from build123d import *

# Parameters (mm, degrees)
BOSS_EXTRUDE1_DEPTH              = 5
MAINSKETCH_19_W                  = 18
MAINSKETCH_19_H                  = 18
BOSS_EXTRUDE2_DEPTH              = 5
CUT_EXTRUDE1_START               = 9
SKETCH1_R                        = 2.5
CUT_EXTRUDE1_DEPTH               = 13
SKETCH2_W                        = 1
SKETCH2_H                        = 3
CUT_EXTRUDE2_DEPTH               = 6
MIRROR2_COPY_1_SKETCH_W          = 1
MIRROR2_COPY_1_SKETCH_H          = 3
MIRROR2_COPY_1_DEPTH             = 6
HOLESKETCH_R                     = 4
CUT_EXTRUDE3_DEPTH               = 6
CUT_EXTRUDE3_DEPTH_BACK          = 2
CUT_EXTRUDE4_DEPTH               = 3
SCHNITT_LINEAR_AUSTRAGEN2_DEPTH  = 2.5
SKIZZE3_R                        = 1.75
SCHNITT_LINEAR_AUSTRAGEN3_DEPTH  = 11
SKIZZE4_R                        = 1.75
SCHNITT_LINEAR_AUSTRAGEN4_DEPTH  = 1.5
SKIZZE6_R                        = 1.75
SCHNITT_LINEAR_AUSTRAGEN6_DEPTH  = 11
SKIZZE7_R                        = 1.75
SCHNITT_LINEAR_AUSTRAGEN7_DEPTH  = 2.5
SKIZZE8_R                        = 1.75
SCHNITT_LINEAR_AUSTRAGEN8_DEPTH  = 11
SKIZZE9_R                        = 1.75
SCHNITT_LINEAR_AUSTRAGEN10_DEPTH = 2.5


with BuildPart() as part:
    # mainSketch → Boss-Extrude1 (new body)
    with BuildSketch(Plane(origin=(0, 0, 0), x_dir=(1, 0, 0), z_dir=(0, 1, 0))):
        with BuildLine():
            ThreePointArc((-18.215390309, 53), (-32.07179677, 53), (-39, 41))
            Line((-39, 41), (-39, -41))
            ThreePointArc((-39, -41), (-32.07179677, -53), (-18.215390309, -53))
            Line((-18.215390309, -53), (31.145825623, -24.501288694))
            ThreePointArc((31.145825623, -24.501288694), (45.291651246, 0), (31.145825623, 24.501288694))
            Line((31.145825623, 24.501288694), (-18.215390309, 53))
        make_face()
        Polygon((-9, -13.55), (-9, 4.45), (-9, 8.45), (9, 8.45), (9, 4.45), (9, -13.55), (9, -17.55), (-9, -17.55), align=None, mode=Mode.SUBTRACT)
    extrude(amount=BOSS_EXTRUDE1_DEPTH)

    # mainSketch_19 → Boss-Extrude2 (add)
    with BuildSketch(Plane(origin=(0, 0, 0), x_dir=(1, 0, 0), z_dir=(0, 1, 0))):
        with BuildLine():
            ThreePointArc((-18.215390309, 53), (-32.07179677, 53), (-39, 41))
            Line((-39, 41), (-39, -41))
            ThreePointArc((-39, -41), (-32.07179677, -53), (-18.215390309, -53))
            Line((-18.215390309, -53), (31.145825623, -24.501288694))
            ThreePointArc((31.145825623, -24.501288694), (45.291651246, 0), (31.145825623, 24.501288694))
            Line((31.145825623, 24.501288694), (-18.215390309, 53))
        make_face()
        with Locations((0, -4.55)):
            Rectangle(MAINSKETCH_19_W, MAINSKETCH_19_H, mode=Mode.SUBTRACT)
    extrude(amount=-BOSS_EXTRUDE2_DEPTH)

    # Sketch1 → Cut-Extrude1 (cut, symmetric)
    with BuildSketch(Plane(origin=(0, 0, 13.55), x_dir=(-1, 0, 0), z_dir=(0, 0, -1)).offset(CUT_EXTRUDE1_START)):
        Circle(SKETCH1_R)
    extrude(amount=CUT_EXTRUDE1_DEPTH, both=True, mode=Mode.SUBTRACT)

    # Sketch2 → Cut-Extrude2 (cut, through all)
    with BuildSketch(Plane(origin=(0, 0, 0), x_dir=(1, 0, 0), z_dir=(0, 1, 0))):
        with Locations((5, -15.55)):
            Rectangle(SKETCH2_W, SKETCH2_H)
    cut_extrude2 = extrude(amount=-CUT_EXTRUDE2_DEPTH, mode=Mode.SUBTRACT)

    # Mirror1: Cut-Extrude2 across plane
    add(cut_extrude2.mirror(Plane(origin=(0, 0, 0), x_dir=(0, 0, 1), z_dir=(1, 0, 0))), mode=Mode.SUBTRACT)

    # Mirror2: Cut-Extrude2 across plane
    add(cut_extrude2.mirror(Plane(origin=(0, 0, 4.55), x_dir=(1, 0, 0), z_dir=(0, 0, -1))), mode=Mode.SUBTRACT)

    # Mirror2 copy 1 sketch → Mirror2 copy 1 (cut, through all)
    with BuildSketch(Plane(origin=(0, 0, 9.1), x_dir=(-1, 0, 0), z_dir=(0, 1, 0))):
        with Locations((5, -15.55)):
            Rectangle(MIRROR2_COPY_1_SKETCH_W, MIRROR2_COPY_1_SKETCH_H)
    extrude(amount=-MIRROR2_COPY_1_DEPTH, mode=Mode.SUBTRACT)

    # holeSketch → Cut-Extrude3 (cut, two sides)
    with BuildSketch(Plane.XZ) as cut_extrude3_sk:
        with Locations(Location((29.25, -15.5, 0), (0, 0, 270))):  # turned: the seam where the file's is
            Circle(HOLESKETCH_R)
        with Locations(Location((-2.443479184, 27.5, 0), (0, 0, 270))):  # turned: the seam where the file's is
            Circle(HOLESKETCH_R)
        with Locations(Location((-29.6, -18.5, 0), (0, 0, 270))):  # turned: the seam where the file's is
            Circle(HOLESKETCH_R)
    extrude(amount=CUT_EXTRUDE3_DEPTH, mode=Mode.SUBTRACT)
    extrude(cut_extrude3_sk.sketch, amount=-CUT_EXTRUDE3_DEPTH_BACK, mode=Mode.SUBTRACT)

    # Sketch3 → Cut-Extrude4 (cut, symmetric)
    with BuildSketch(Plane(origin=(0, 0, 0), x_dir=(1, 0, 0), z_dir=(0, 1, 0))):
        with BuildLine():
            Line((-29.6, 26.5), (-39, 26.5))
            Line((-39, 26.5), (-39.6, 26.5))
            Line((-39.6, 26.5), (-39.6, -6.5))
            Line((-39.6, -6.5), (-37.6, -6.5))
            Line((-37.6, -6.5), (-21.6, -6.5))
            Line((-21.6, -6.5), (-21.6, 18.5))
            ThreePointArc((-21.6, 18.5), (-23.943145751, 24.156854249), (-29.6, 26.5))
        make_face()
        with BuildLine():
            Line((4.484724046, -23.5), (11.583570163, -35.79556215))
            Line((11.583570163, -35.79556215), (-8.960116539, -56.33889432))
            Line((-8.960116539, -56.33889432), (-14.464495813, -50.834420053))
            Line((-14.464495813, -50.834420053), (-25.778106688, -39.520613931))
            Line((-25.778106688, -39.520613931), (-8.100284622, -21.843096939))
            ThreePointArc((-8.100284622, -21.843096939), (-1.399235427, -19.568445614), (4.484724046, -23.5))
        make_face()
        with BuildLine():
            Line((40.858217841, 16.978745932), (35.413092194, 10.399382918))
            ThreePointArc((35.413092194, 10.399382918), (30.548118213, 7.606021972), (25.044818187, 8.694381298))
            Line((25.044818187, 8.694381298), (3.777259743, 21.835574464))
            Line((3.777259743, 21.835574464), (12.187623369, 35.446811868))
            Line((12.187623369, 35.446811868), (14.338041609, 38.927024434))
            Line((14.338041609, 38.927024434), (40.858217841, 16.978745932))
        make_face()
    extrude(amount=CUT_EXTRUDE4_DEPTH, both=True, mode=Mode.SUBTRACT)

    # Skizze2 → Schnitt-Linear austragen2 (cut, symmetric)
    with BuildSketch(Plane(origin=(0, 0, 0), x_dir=(1, 0, 0), z_dir=(0, 1, 0))):
        with BuildLine():
            ThreePointArc((45.291651246, 0), (45.130303789, 3.017207151), (44.648101747, 6))
            Line((44.648101747, 6), (25.291651246, 6))
            Line((25.291651246, 6), (25.291651246, -6))
            Line((25.291651246, -6), (44.648101747, -6))
            ThreePointArc((44.648101747, -6), (45.130303789, -3.017207151), (45.291651246, 0))
        make_face()
    extrude(amount=SCHNITT_LINEAR_AUSTRAGEN2_DEPTH, both=True, mode=Mode.SUBTRACT)

    # Skizze3 → Schnitt-Linear austragen3 (cut, through all)
    with BuildSketch(Plane(origin=(0, 5, 0), x_dir=(1, 0, 0), z_dir=(0, 1, 0))):
        with Locations(Location((31.291651246, 0, 0), (0, 0, 270))):  # turned: the seam where the file's is
            Circle(SKIZZE3_R)
    extrude(amount=-SCHNITT_LINEAR_AUSTRAGEN3_DEPTH, mode=Mode.SUBTRACT)

    # Skizze4 → Schnitt-Linear austragen4 (cut)
    with BuildSketch(Plane.XZ.offset(5)):
        Polygon((34.291651246, 1.732050808), (31.291651246, 3.464101615), (28.291651246, 1.732050808), (28.291651246, -1.732050808), (31.291651246, -3.464101615), (34.291651246, -1.732050808), align=None)
        with Locations(Location((31.291651246, 0, 0), (0, 0, 90))):  # turned: the seam where the file's is
            Circle(SKIZZE4_R, mode=Mode.SUBTRACT)
    extrude(amount=-SCHNITT_LINEAR_AUSTRAGEN4_DEPTH, mode=Mode.SUBTRACT)

    # Skizze6 → Schnitt-Linear austragen6 (cut, through all)
    with BuildSketch(Plane(origin=(0, 5, 0), x_dir=(1, 0, 0), z_dir=(0, 1, 0))):
        with Locations(Location((20, -5, 0), (0, 0, 270))):  # turned: the seam where the file's is
            Circle(SKIZZE6_R)
        with BuildLine():
            Line((18.25, 4), (18.25, 8))
            ThreePointArc((18.25, 8), (20, 9.75), (21.75, 8))
            Line((21.75, 8), (21.75, 4))
            ThreePointArc((21.75, 4), (20, 2.25), (18.25, 4))
        make_face()
    extrude(amount=-SCHNITT_LINEAR_AUSTRAGEN6_DEPTH, mode=Mode.SUBTRACT)

    # Skizze7 → Schnitt-Linear austragen7 (cut)
    with BuildSketch(Plane.XZ.offset(5)):
        Polygon((23, 3.267949192), (23, 6.732050808), (20, 8.464101615), (17, 6.732050808), (17, 3.267949192), (20, 1.535898385), align=None)
        with Locations(Location((20, 5, 0), (0, 0, 90))):  # turned: the seam where the file's is
            Circle(SKIZZE7_R, mode=Mode.SUBTRACT)
        with BuildLine():
            Line((17, -2.267949192), (17, -5.732050808))
            Line((17, -5.732050808), (17.464101615, -6))
            Line((17.464101615, -6), (18.25, -5.546261356))
            Line((18.25, -5.546261356), (18.25, -4))
            ThreePointArc((18.25, -4), (20, -2.25), (21.75, -4))
            Line((21.75, -4), (21.75, -5.546261356))
            Line((21.75, -5.546261356), (22.535898385, -6))
            Line((22.535898385, -6), (23, -5.732050808))
            Line((23, -5.732050808), (23, -2.267949192))
            Line((23, -2.267949192), (20, -0.535898385))
            Line((20, -0.535898385), (17, -2.267949192))
        make_face()
        with BuildLine():
            Line((17.464101615, -6), (17, -6.267949192))
            Line((17, -6.267949192), (17, -9.732050808))
            Line((17, -9.732050808), (20, -11.464101615))
            Line((20, -11.464101615), (23, -9.732050808))
            Line((23, -9.732050808), (23, -6.267949192))
            Line((23, -6.267949192), (22.535898385, -6))
            Line((22.535898385, -6), (21.75, -6.453738644))
            Line((21.75, -6.453738644), (21.75, -8))
            ThreePointArc((21.75, -8), (20, -9.75), (18.25, -8))
            Line((18.25, -8), (18.25, -6.453738644))
            Line((18.25, -6.453738644), (17.464101615, -6))
        make_face()
        Polygon((17.464101615, -6), (17, -5.732050808), (17, -6.267949192), align=None)
        Polygon((18.25, -5.546261356), (17.464101615, -6), (18.25, -6.453738644), align=None)
        Polygon((21.75, -5.546261356), (21.75, -6.453738644), (22.535898385, -6), align=None)
        Polygon((23, -6.267949192), (23, -5.732050808), (22.535898385, -6), align=None)
    extrude(amount=-SCHNITT_LINEAR_AUSTRAGEN7_DEPTH, mode=Mode.SUBTRACT)

    # Skizze8 → Schnitt-Linear austragen8 (cut, through all)
    with BuildSketch(Plane(origin=(0, 5, 0), x_dir=(1, 0, 0), z_dir=(0, 1, 0))):
        with Locations(Location((-10, 15.45, 0), (0, 0, 270))):  # turned: the seam where the file's is
            Circle(SKIZZE8_R)
        with Locations(Location((10, -24.55, 0), (0, 0, 270))):  # turned: the seam where the file's is
            Circle(SKIZZE8_R)
    extrude(amount=-SCHNITT_LINEAR_AUSTRAGEN8_DEPTH, mode=Mode.SUBTRACT)

    # Skizze9 → Schnitt-Linear austragen10 (cut)
    with BuildSketch(Plane(origin=(0, -5, 0), x_dir=(1, 0, 0), z_dir=(0, 1, 0))):
        Polygon((-10, 18.914101615), (-13, 17.182050808), (-13, 13.717949192), (-10, 11.985898385), (-7, 13.717949192), (-7, 17.182050808), align=None)
        with Locations(Location((-10, 15.45, 0), (0, 0, 270))):  # turned: the seam where the file's is
            Circle(SKIZZE9_R, mode=Mode.SUBTRACT)
        Polygon((13, -26.282050808), (13, -22.817949192), (10, -21.085898385), (7, -22.817949192), (7, -26.282050808), (10, -28.014101615), align=None)
        with Locations(Location((10, -24.55, 0), (0, 0, 270))):  # turned: the seam where the file's is
            Circle(SKIZZE9_R, mode=Mode.SUBTRACT)
    extrude(amount=SCHNITT_LINEAR_AUSTRAGEN10_DEPTH, mode=Mode.SUBTRACT)


solid = part.part
Geometry check sheet. Reference: the model listing, model coordinates, mm. A direction names the side the tool comes from. Round coordinates to 2 decimals unless told otherwise and drop trailing zeros. Order: outer loops, then holes, each group sorted by start corner. A loop starts at its lowest first (then second) coordinate and runs counter-clockwise, first axis right, second up. Notation, with made-up numbers: M -19,44.25 L 23,44.25 A34 cw 23,74.25 Z; hole C -39,-7.75 d4. An arc over 180 degrees is marked long. Write each question's results on one line, items separated by ' | '. Start each with the question number.
1. Cross-section at C-C on y = -1.25. Give the number of separate pieces and of enclosed holes in the cut face, plus the area to 3 significant figures.
2. Material ranges on L1, parallel to X at y = 4, z = 0; L2, parallel to X at y = -0.75, z = 5; L3, parallel to X at y = -3.55, z = -15.5, recorded low to high. Write a range as from..to.
3. Draft check along X on faces 1 (the face through (7.984, -0.042, 29.562)), 2 (the face through (25.292, 0, 0)), 3 (the face through (-39, 3.4, -0.6)). Enter one of: pulls with the +X half, pulls with the -X half, needs draft (parallel to the pull), parting line crosses it, or undercut.
4. Cross-section at B-B on x = 38. Record the boundary of the cut face in (y, z).
5. Cross-section at A-A on x = 0. Record the boundary of the cut face in (y, z).
6. Set-up check for faces 4 (the face through (17, -4, 5)), 5 (the face through (6, 0, 16)), 6 (the face through (19.96, 1.3, -9.75)), 7 (the face through (-7, -3, 35)), 8 (the face through (37.84, 0.04, -13.33)): record each of +Z, -Z, +X, -X, +Y, -Y from which the full face is reachable in a straight line by a thin tool's end or side.
7. Go/stop test with flat-tipped pins: P1, Ø4, axis at x = 31.29, z = 0, coming from the -Y side; P2, Ø1.5, axis at y = -0.5, z = 35, coming from the +X side; P3, Ø3.5, axis at y = -2.5, z = 15, coming from the +X side. Record where each tip stops, or that it passes through.
Resolved:
1) separate pieces: 1 | enclosed holes: 9 | area: 4,130 mm2
2) L1: -39..-9, 9..29.54, 33.04..45.29 | L2: -21.6..-9, 9..18.25, 21.75..25.29 | L3: -39..-32.25, -26.95..-13, -7..25.25, 33.25..40.67
3) face 1: undercut | face 2: pulls with the +X half | face 3: pulls with the -X half
4) outline: M -5,-18.96 L -3,-18.96 L -3,-13.53 L 3,-13.53 L 3,-18.96 L 5,-18.96 L 5,18.96 L -5,18.96 Z; hole M -2.5,-6 L 2.5,-6 L 2.5,6 L -2.5,6 Z
5) outline: M -5,-42.48 L 5,-42.48 L 5,-8.45 L -2.5,-8.45 L -2.5,-4.45 L -5,-4.45 Z; M -5,13.55 L -2.5,13.55 L -2.5,17.55 L 5,17.55 L 5,42.48 L 3,42.48 L 3,19.88 L -3,19.88 L -3,24.33 L -5,24.33 Z; M -5,30.67 L -3,30.67 L -3,42.48 L -5,42.48 Z
6) face 4: -Y | face 5: +Y | face 6: +Y, -Y | face 7: none | face 8: -Z
7) P1: y = -3.5 | P2: x = 14.26 | P3: x = 42
